from build123d import *

# Parameters (mm, degrees)
BOSS_EXTRUDE1_DEPTH     = 55
CUT_EXTRUDE1_DEPTH      = 56.084783138
CUT_EXTRUDE1_DEPTH_BACK = 56.084783138
SKETCH2_R               = 1.25


with BuildPart() as part:
    # Sketch1 → Boss-Extrude1 (new body)
    with BuildSketch(Plane.XY):
        Polygon((2.309401077, 0), (1.154700538, 2), (-1.154700538, 2), (-2.309401077, 0), (-1.154700538, -2), (1.154700538, -2), align=None)
    extrude(amount=-BOSS_EXTRUDE1_DEPTH)

    # Sketch2 → Cut-Extrude1 (cut, two sides: drawn at the far end of the back side and taken through both)
    with BuildSketch(Plane.XY.offset(-CUT_EXTRUDE1_DEPTH_BACK)):
        Circle(SKETCH2_R)
    extrude(amount=CUT_EXTRUDE1_DEPTH + CUT_EXTRUDE1_DEPTH_BACK, mode=Mode.SUBTRACT)


solid = part.part
Verification items for the finished model (mm, model axes). Coordinates: 2 decimals unless noted, no trailing zeros. Order: outer loops, then holes, each group sorted by start corner. A loop starts at its lowest first (then second) coordinate and runs counter-clockwise, first axis right, second up.
Item 1: Release check for a two-part mould opening along X. For faces 1 (the face through (-0.27, -1.22, -27.88)), 2 (the face through (0, 2, -27)), 3 (the face through (1.724, -1.014, -27.115)) record: +X half, -X half, draft (parallel to the pull), parting line (faces both ways), or undercut.
Filled in:
face 1: undercut
face 2: draft
face 3: +X half
Item 2: Material ranges on L1, parallel to X at y = 0, z = -43; L2, parallel to Y at x = 0, z = -33.5; L3, parallel to X at y = 0.6, z = -6.5, recorded low to high.
Filled in:
L1: x = -2.31 to -1.25, 1.25 to 2.31
L2: y = -2 to -1.25, 1.25 to 2
L3: x = -1.96 to -1.1, 1.1 to 1.96
Item 3: Section check B-B, the plane z = -44.5. Enter the section's corners in (x, y), then the cut area to 3 significant figures.
Filled in:
outline: (-2.31, 0) - (-1.15, -2) - (1.15, -2) - (2.31, 0) - (1.15, 2) - (-1.15, 2) - close; hole circle Ø2.5 at (0, 0)
area: 8.95 mm2
Item 4: Section check A-A, the plane x = 0. Enter the section's corners in (y, z).
Filled in:
outline: (-2, -55) - (-1.25, -55) - (-1.25, 0) - (-2, 0) - close; (1.25, -55) - (2, -55) - (2, 0) - (1.25, 0) - close
